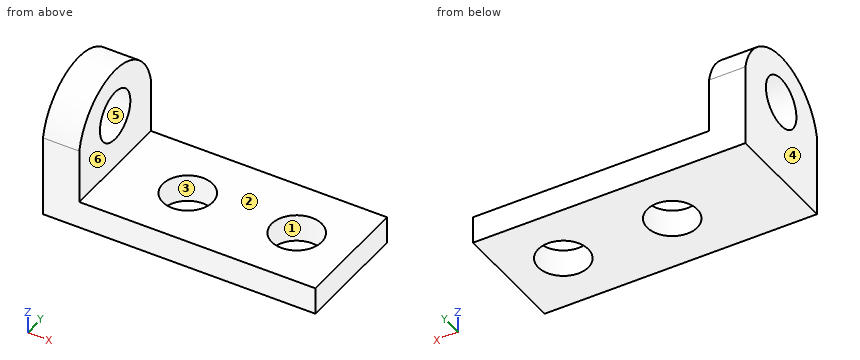
```python
from build123d import *

# Parameters (mm, degrees)
F0_W     = 190.5
F0_H     = 82.55
F0_R     = 17.526
F1_DEPTH = 19.05
F2_W     = 82.55
F2_H     = 57.15
F3_DEPTH = 25.4
F4_R     = 17.526
F5_DEPTH = 25.4


with BuildPart() as f1:
    # F0 (on Top) → F1 (new body)
    with BuildSketch(Plane.XY):
        with Locations((-30.811098, 9.839004)):
            Rectangle(F0_W, F0_H)
        with Locations((-49.861098, 9.839004)):
            Circle(F0_R, mode=Mode.SUBTRACT)
        with Locations((26.338902, 9.839004)):
            Circle(F0_R, mode=Mode.SUBTRACT)
    extrude(amount=-F1_DEPTH)

    # F2 (on face) → F3 (join)
    with BuildSketch(Plane(origin=(-126.061098, 0, 0), x_dir=(0, -1, 0), z_dir=(-1, 0, 0))):
        with Locations((-9.839004, 9.525)):
            Rectangle(F2_W, F2_H)
        with BuildLine():
            ThreePointArc((31.435996, 38.1), (-9.839004, 72.125149), (-51.114004, 38.1))
            Line((-51.114004, 38.1), (31.435996, 38.1))
        make_face()
    extrude(amount=-F3_DEPTH)

    # F4 (on face) → F5 (cut)
    with BuildSketch(Plane(origin=(-126.061098, 0, 0), x_dir=(0, -1, 0), z_dir=(-1, 0, 0))):
        with Locations((-9.839004, 38.1)):
            Circle(F4_R)
    extrude(amount=-F5_DEPTH, mode=Mode.SUBTRACT)


solid = f1.part
```
The model under review builds one solid part; all positions refer to its coordinate system, in mm. Face numbers are marked on the shaded views. A direction names the side the tool comes from. Round coordinates to 2 decimals unless told otherwise and drop trailing zeros. Loops run counter-clockwise (first coordinate to the right, second up) from the corner with the lowest first, then second, coordinate; pieces in that order, holes last. Notation, with made-up numbers: (54, 18) -> (93, 18) arc R21 cw to (93, 23) -> close; hole circle Ø9 at (67.5, 49). An arc over 180 degrees is marked (long way). Answer as a JSON object with one key per item and string values. Group by question number.
1) We need section B-B on y = 25.5. Write out the cut boundary in (x, z), then the cut area to 3 significant figures.
2) For pin 1 Ø8 at (x, y) = (-33.5, 11.5) entering from +Z; pin 2 Ø6 at (y, z) = (38, 31.5) entering from +X, all flat-tipped, find the tip position at first contact; note any pin that passes through.
3) Mouldability with a two-part tool opening along X and no side actions: class the marked faces 1, 2, 3 and 4 as released by +X, released by -X, zero draft, split by the parting line, or undercut.
4) We need section C-C on x = -56. Write out the cut boundary in (y, z), then the cut area to 3 significant figures.
5) For the marked faces 5 and 6, list the 3-axis set-ups (+Z, -Z, +X, -X, +Y, -Y) from which the entire face can be reached by the end or side of a thin tool; tool diameter is ignored.
6) We need section D-D on x = -7. Write out the cut boundary in (y, z).
7) We need section A-A on z = 28. Write out the cut boundary in (x, y).
8) For line 1 (X direction, y = 10.5, z = -7.5); line 2 (Y direction, x = -114, z = 38); line 3 (Z direction, x = -14.5, y = -20), list the stretches that pass through material, from the lowest coordinate up. Write a range as [from, to].
Result set:
{
 "1": {"outline": "(-126.06, -19.05) -> (-57.73, -19.05) -> (-57.73, 0) -> (-100.66, 0) -> (-100.66, 30.23) -> (-126.06, 30.23) -> close; (-126.06, 45.97) -> (-100.66, 45.97) -> (-100.66, 69.1) -> (-126.06, 69.1) -> close; (-41.99, -19.05) -> (18.47, -19.05) -> (18.47, 0) -> (-41.99, 0) -> close; (34.21, -19.05) -> (64.44, -19.05) -> (64.44, 0) -> (34.21, 0) -> close", "area": "4,390 mm²"},
 "2": {"pin 1": "z = 0", "pin 2": "x = -100.66"},
 "3": {"face 1": "undercut", "face 2": "zero draft", "face 3": "undercut", "face 4": "released by -X"},
 "4": {"outline": "(-31.44, -19.05) -> (-6.58, -19.05) -> (-6.58, 0) -> (-31.44, 0) -> close; (26.25, -19.05) -> (51.11, -19.05) -> (51.11, 0) -> (26.25, 0) -> close", "area": "947 mm²"},
 "5": {"face 5": "+X, -X", "face 6": "+Z, +X, +Y, -Y"},
 "6": {"outline": "(-31.44, -19.05) -> (51.11, -19.05) -> (51.11, 0) -> (-31.44, 0) -> close"},
 "7": {"outline": "(-126.06, -31.44) -> (-100.66, -31.44) -> (-100.66, -4.48) -> (-126.06, -4.48) -> close; (-126.06, 24.16) -> (-100.66, 24.16) -> (-100.66, 51.11) -> (-126.06, 51.11) -> close"},
 "8": {"line 1": "[-126.06, -67.37], [-32.35, 8.83], [43.85, 64.44]", "line 2": "[-31.44, -7.69], [27.36, 51.11]", "line 3": "[-19.05, 0]"}
}
